Design review of the part shown in the three views and the two pictorial views. Dimensions are in mm from the part's minimum x, y and z. Round coordinates to 2 decimals unless told otherwise and drop trailing zeros. Order: outer loops, then holes, each group sorted by start corner. A loop starts at its lowest first (then second) coordinate and runs counter-clockwise, first axis right, second up.
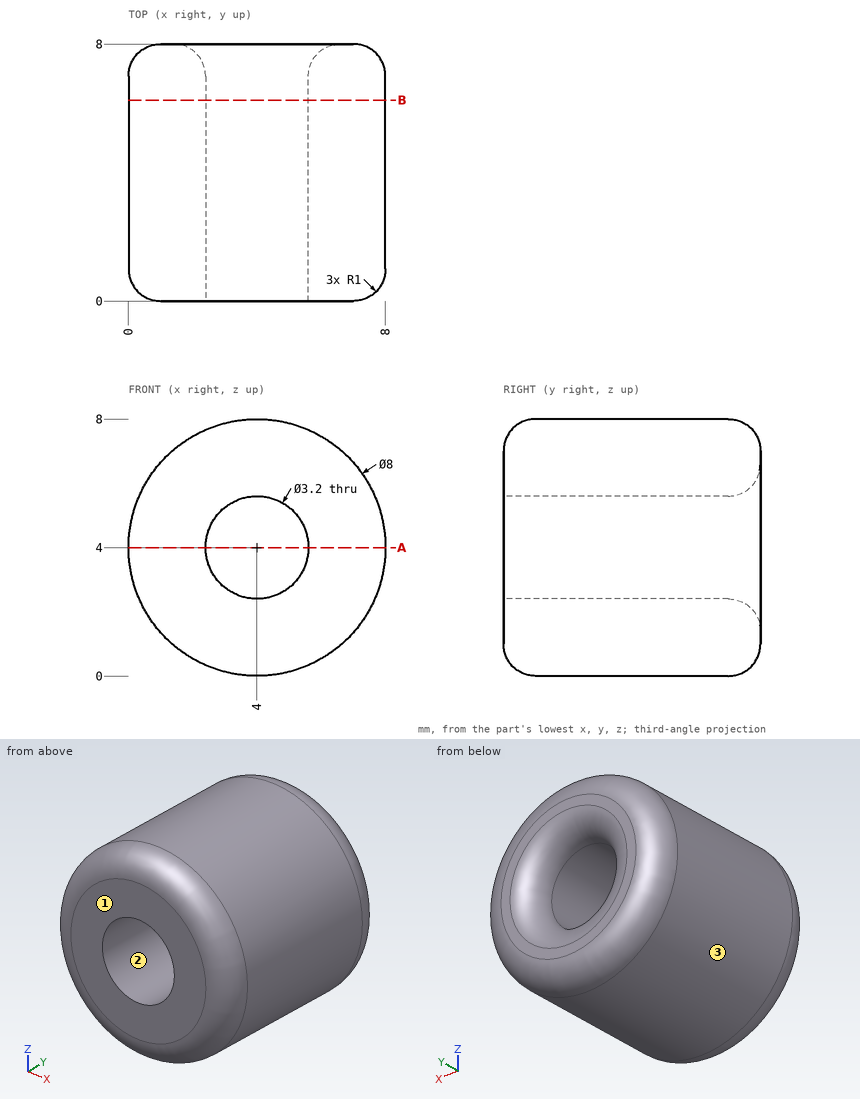
1) Take a section at B-B on y = 6.25. Give the boundary of the cut face in (x, z), plus the area to 3 significant figures.
Results:
outline: circle Ø8 at (4, 4); hole circle Ø3.2 at (4, 4)
area: 42.2 mm2
2) The part is to be moulded in two halves that separate along Z. For the marked faces 1, 2 and 3, say which applies: released by +Z, released by -Z, zero draft, split by the parting line, or undercut.
Results:
face 1: zero draft
face 2: undercut
face 3: split by the parting line
3) To check wall thickness, follow line 1 along X through (y, z) = (4.75, 4); line 2 along Y through (x, z) = (3.5, 1.5). State the ranges of each line that lie inside material, in increasing order.
Results:
line 1: x = 0 to 2.4, 5.6 to 8
line 2: y = 0 to 8
4) Clearance check with flat-ended pins moving along their axes: P1, Ø3, axis at y = 6, z = 5, coming from the +X side; P2, Ø3, axis at x = 1, y = 4.5, coming from the -Z side; P3, Ø2, axis at y = 4, z = 7, coming from the -X side; P4, Ø1, axis at x = 5, z = 4, coming from the +Y side (3 decimals). State where each tip first meets the part, or that it passes through.
Results:
P1: stops at x = 8
P2: stops at z = 0.29
P3: stops at x = 0.54
P4: passes through
5) Take a section at A-A on z = 4. Give the boundary of the cut face in (x, y), plus the area to 3 significant figures.
Results:
outline: (0, 1) arc R1 ccw to (1, 0) - (2.4, 0) - (2.4, 7) arc R1 ccw to (1.4, 8) - (1, 8) arc R1 ccw to (0, 7) - close; (5.6, 0) - (7, 0) arc R1 ccw to (8, 1) - (8, 7) arc R1 ccw to (7, 8) - (6.6, 8) arc R1 ccw to (5.6, 7) - close
area: 37.1 mm2
